from build123d import *

# Parameters (mm, degrees)
SKETCH1_W           = 10
SKETCH1_H           = 40
BOSS_EXTRUDE1_DEPTH = 10
CUT_EXTRUDE1_REACH  = 44.426
SKETCH2_R           = 2
SKETCH3_W           = 10
SKETCH3_H           = 10
BOSS_EXTRUDE2_DEPTH = 20
CUT_EXTRUDE2_REACH  = 52.99
SKETCH4_R           = 2
SKETCH5_R           = 2
CUT_EXTRUDE3_DEPTH  = 51.990195136
FILLET1_R           = 5


with BuildPart() as part:
    # Sketch1 → Boss-Extrude1 (new body)
    with BuildSketch(Plane.XY):
        with Locations((5, 20)):
            Rectangle(SKETCH1_W, SKETCH1_H)
    extrude(amount=BOSS_EXTRUDE1_DEPTH)

    # Sketch2 → Cut-Extrude1 (cut, up to next)
    with BuildSketch(Plane(origin=(10, 0, 0), x_dir=(0, 0, -1), z_dir=(1, 0, 0)), mode=Mode.PRIVATE) as cut_extrude1_sk1:
        with Locations((-5, 5)):
            Circle(SKETCH2_R)
    cut_extrude1_tool1 = extrude(cut_extrude1_sk1.sketch, amount=-CUT_EXTRUDE1_REACH, mode=Mode.PRIVATE) & part.part
    add(cut_extrude1_tool1.solids().sort_by_distance((10, 5, 5))[0], mode=Mode.SUBTRACT)

    # Sketch3 → Boss-Extrude2 (add)
    with BuildSketch(Plane.XY.offset(10)):
        with Locations((5, 25)):
            Rectangle(SKETCH3_W, SKETCH3_H)
    extrude(amount=BOSS_EXTRUDE2_DEPTH)

    # Sketch4 → Cut-Extrude2 (cut, up to next)
    with BuildSketch(Plane.ZY, mode=Mode.PRIVATE) as cut_extrude2_sk1:
        with Locations((25, 25)):
            Circle(SKETCH4_R)
    cut_extrude2_tool1 = extrude(cut_extrude2_sk1.sketch, amount=-CUT_EXTRUDE2_REACH, mode=Mode.PRIVATE) & part.part
    add(cut_extrude2_tool1.solids().sort_by_distance((0, 25, 25))[0], mode=Mode.SUBTRACT)

    # Sketch5 → Cut-Extrude3 (cut, through all)
    with BuildSketch(Plane.ZY):
        with Locations((5, 25)):
            Circle(SKETCH5_R)
    extrude(amount=-CUT_EXTRUDE3_DEPTH, mode=Mode.SUBTRACT)

    # Fillet1
    fillet1_edges = [part.edges().sort_by_distance(p)[0] for p in [
        (5, 0, 0),
        (5, 0, 10),
    ]]
    fillet(fillet1_edges, radius=FILLET1_R - 0.0001)  # a hair under: the kernel refuses the full size


solid = part.part
Verification items for the finished model (mm, model axes). A direction names the side the tool comes from. Give positions to 0.01 mm unless a question says otherwise; leave off trailing zeros. Write each loop counter-clockwise with the first axis right and the second up, starting at its lowest first coordinate (ties: lowest second). Pieces come first, ordered by that corner, then holes. Notation, with made-up numbers: M 55.5,-14.75 L 60.5,-14.75 A26 ccw 60.5,11.25 Z; hole C 41,-35.75 d6. An arc over 180 degrees is marked long. Put each result on its own line as item: value. Start each with the question number.
1. Set-up check for faces 1 (the face through (5, 20, 20)), 2 (the face through (5, 5, 7)), 3 (the face through (5, 35, 10)): record each of +Z, -Z, +X, -X, +Y, -Y from which the full face is reachable in a straight line by a thin tool's end or side.
2. Draft check along Z on faces 4 (the face through (5, 30, 20)), 5 (the face through (4.9, 23.8, 23.4)), 6 (the face through (5, 23, 0)). Enter one of: +Z half, -Z half, draft (parallel to the pull), parting line (faces both ways), or undercut.
3. Section check D-D (y = 32). Record the cut outline in (x, z), and give its area (3 significant figures).
4. Scan lines: line 1 along Y through (x, z) = (5.5, 5); line 2 along Y through (x, z) = (6, 25); line 3 along Z through (x, y) = (3.5, 17). Record each from-to range of solid material in increasing order. Write a range as [from, to].
5. Section check A-A (y = 25). Record the cut outline in (x, z).
6. Go/stop test with flat-tipped pins: pin 1 Ø4.5 at (y, z) = (25, 5) entering from +X; pin 2 Ø3 at (x, y) = (7, 14.5) entering from +Z; pin 3 Ø3.5 at (y, z) = (5, 5) entering from +X (1 decimal). Record where each tip stops, or that it passes through.
7. Section check C-C (z = 22). Record the cut outline in (x, y), and give its area (3 significant figures).
8. Section check B-B (x = 3.5). Give the number of separate pieces and of enclosed holes in the cut face, and give its area (3 significant figures).
Answer list:
1. face 1: +Z, +X, -X, -Y
1. face 2: +X, -X
1. face 3: +Z, +X, -X, +Y
2. face 4: draft
2. face 5: undercut
2. face 6: -Z half
3. outline: M 0,0 L 10,0 L 10,10 L 0,10 Z
3. area: 100 mm2
4. line 1: [0, 3], [7, 23], [27, 40]
4. line 2: [20, 23], [27, 30]
4. line 3: [0, 10]
5. outline: M 0,0 L 10,0 L 10,3 L 0,3 Z; M 0,7 L 10,7 L 10,23 L 0,23 Z; M 0,27 L 10,27 L 10,30 L 0,30 Z
6. pin 1: x = 10
6. pin 2: z = 10
6. pin 3: through
7. outline: M 0,20 L 10,20 L 10,30 L 0,30 Z
7. area: 100 mm2
8. separate pieces: 1
8. enclosed holes: 3
8. area: 552 mm2
